```python
from build123d import *

# Parameters (mm, degrees)
F0_R      = 13.9889248678
F1_DEPTH  = 25.4
F2_SIZE   = 12.69999
F3_W      = 76.2
F3_H      = 76.2
F4_DEPTH  = 76.2
F5_W      = 25.4
F5_H      = 25.4
F7_DEPTH  = 76.2
F8_W      = 25.4
F8_H      = 25.4
F9_DEPTH  = 76.2
F10_W     = 25.4
F10_H     = 25.4
F11_DEPTH = 76.2


# Not quite as in the source:
# - a fillet or chamfer is up to 0.001 mm smaller than in the source, because OpenCascade refuses the exact size


with BuildPart() as f1:
    # F0 (on Top) → F1 (new body)
    with BuildSketch(Plane.XY):
        with Locations((-42.8192056715, -23.4777331352)):
            Circle(F0_R)
    extrude(amount=F1_DEPTH)

    # F2 (size 12.7 in the source; OpenCascade refuses exactly that, so slightly less here)
    f2_edges = [f1.edges().sort_by_distance(p)[0] for p in [
        (-28.830281, -23.477733, 12.7),
        (-56.808131, -23.477733, 0),
        (-56.808131, -23.477733, 25.4),
    ]]
    chamfer(f2_edges, length=F2_SIZE)


with BuildPart() as f4:
    # F3 (on Top) → F4 (new body)
    with BuildSketch(Plane.XY):
        with Locations((54.4739740274, 3.576669842)):
            Rectangle(F3_W, F3_H)
    extrude(amount=F4_DEPTH)

    # F5 (on face) → F7 (cut)
    with BuildSketch(Plane.XZ.offset(34.523330158)):
        with Locations((29.0739740274, 63.5)):
            Rectangle(F5_W, F5_H)
        with Locations((79.8739740274, 63.5)):
            Rectangle(F5_W, F5_H)
        with Locations((79.8739740274, 12.7)):
            Rectangle(F5_W, F5_H)
        with Locations((29.0739740274, 12.7)):
            Rectangle(F5_W, F5_H)
    extrude(amount=-F7_DEPTH, mode=Mode.SUBTRACT)

    # F8 (on face) → F9 (cut)
    with BuildSketch(Plane.YZ.offset(92.5739740274)):
        with Locations((-21.823330158, 12.7)):
            Rectangle(F8_W, F8_H)
        with Locations((-21.823330158, 63.5)):
            Rectangle(F8_W, F8_H)
        with Locations((28.976669842, 63.5)):
            Rectangle(F8_W, F8_H)
        with Locations((28.976669842, 12.7)):
            Rectangle(F8_W, F8_H)
    extrude(amount=-F9_DEPTH, mode=Mode.SUBTRACT)

    # F10 (on face) → F11 (cut)
    with BuildSketch(Plane.XY.offset(50.8)):
        with Locations((79.8739740274, -21.823330158)):
            Rectangle(F10_W, F10_H)
        with Locations((79.8739740274, 28.976669842)):
            Rectangle(F10_W, F10_H)
        with Locations((29.0739740274, 28.976669842)):
            Rectangle(F10_W, F10_H)
        with Locations((29.0739740274, -21.823330158)):
            Rectangle(F10_W, F10_H)
    extrude(amount=-F11_DEPTH, mode=Mode.SUBTRACT)


solid = f4.part
```
CAD build for the part. Positions are in the model's coordinates, mm. A direction names the side the tool comes from. Round coordinates to 2 decimals unless told otherwise and drop trailing zeros. Order: outer loops, then holes, each group sorted by start corner. A loop starts at its lowest first (then second) coordinate and runs counter-clockwise, first axis right, second up.
Item 1: Saw through at A-A on x = 59. Write the cut outline in (y, z), then the cut area to 3 significant figures.
Item 2: Saw through at B-B on y = 12.5. Write the cut outline in (x, z).
Item 3: Pin check, flat tips, straight feed: pin 1 (12 mm diameter, centred on x = 81, z = 20.5, fed in from -Y); pin 2 (7.5 mm diameter, centred on x = 80.5, y = 8.5, fed in from -Z); pin 3 (7.5 mm diameter, centred on x = 85.5, y = 4, fed in from +Z); pin 4 (6 mm diameter, centred on x = 36, z = 19, fed in from +Y). Stop position of each tip, or through.
Item 4: Saw through at C-C on z = 63. Write the cut outline in (x, y).
Item 5: Tool access for faces 1 (the face through (54, -22, 25.4)), 2 (the face through (41.774, 3, 63)), 3 (the face through (80, 3, 25.4)), 4 (the face through (67.174, 29, 38)): list every direction of +Z, -Z, +X, -X, +Y, -Y with a clear straight run to the whole face (end or side of a thin tool).
Item 6: Saw through at D-D on x = 77. Write the cut outline in (y, z).
Item 7: Probe line 1 along Y through (x, z) = (55, 19.5); line 2 along Z through (x, y) = (58, -27.5); line 3 along X through (y, z) = (-10, 30). List the from-to ranges inside material, lowest first.
Reported:
1. outline: (-34.52, 25.4) - (-9.12, 25.4) - (-9.12, 0) - (16.28, 0) - (16.28, 25.4) - (41.68, 25.4) - (41.68, 50.8) - (16.28, 50.8) - (16.28, 76.2) - (-9.12, 76.2) - (-9.12, 50.8) - (-34.52, 50.8) - close
1. area: 3,230 mm2
2. outline: (16.37, 25.4) - (41.77, 25.4) - (41.77, 0) - (67.17, 0) - (67.17, 25.4) - (92.57, 25.4) - (92.57, 50.8) - (67.17, 50.8) - (67.17, 76.2) - (41.77, 76.2) - (41.77, 50.8) - (16.37, 50.8) - close
3. pin 1: stops at y = -9.12
3. pin 2: stops at z = 25.4
3. pin 3: stops at z = 50.8
3. pin 4: passes through
4. outline: (41.77, -9.12) - (67.17, -9.12) - (67.17, 16.28) - (41.77, 16.28) - close
5. face 1: -Z, +X, -X, -Y
5. face 2: +Z, -X, +Y, -Y
5. face 3: -Z, +X, +Y, -Y
5. face 4: +Z, -Z, +X, +Y
6. outline: (-9.12, 25.4) - (16.28, 25.4) - (16.28, 50.8) - (-9.12, 50.8) - close
7. line 1: y = -9.12 to 16.28
7. line 2: z = 25.4 to 50.8
7. line 3: x = 41.77 to 67.17
